```python
from build123d import *

# Parameters (mm, degrees)
SKETCH1_R           = 3
BOSS_EXTRUDE1_DEPTH = 101.6
BOSS_EXTRUDE2_START = 3.175
SKETCH3_R           = 1.0795
BOSS_EXTRUDE2_DEPTH = 3.175


with BuildPart() as part:
    # Sketch1 → Boss-Extrude1 (new body)
    with BuildSketch(Plane(origin=(0, 0, 0), x_dir=(1, 0, 0), z_dir=(0, 1, 0))):
        with Locations(Location((0, 0, 0), (0, 0, 270))):
            Circle(SKETCH1_R)
    extrude(amount=BOSS_EXTRUDE1_DEPTH)

    # Sketch3 → Boss-Extrude2 (add)
    with BuildSketch(Plane.XZ.offset(BOSS_EXTRUDE2_START)):
        with BuildLine():
            Line((-3, 0), (-3, 9.7))
            Line((-3, 9.7), (1.445, 9.7))
            Line((1.445, 9.7), (9.7, 1.445))
            Line((9.7, 1.445), (9.7, -3))
            Line((9.7, -3), (0, -3))
            ThreePointArc((0, -3), (-2.121320344, -2.121320344), (-3, 0))
        make_face()
        with Locations(Location((0.048, 6.34981858, 0), (0, 0, 270))):
            Circle(SKETCH3_R, mode=Mode.SUBTRACT)
        with Locations(Location((6.34981858, 0.048, 0), (0, 0, 270))):
            Circle(SKETCH3_R, mode=Mode.SUBTRACT)
    extrude(amount=-BOSS_EXTRUDE2_DEPTH)


solid = part.part
```
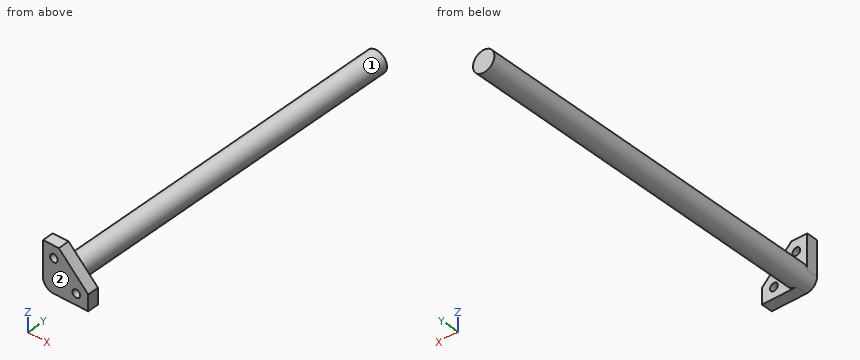
Part model, mm, in its own coordinate system. Face numbers are marked on the shaded views. A direction names the side the tool comes from. Round coordinates to 2 decimals unless told otherwise and drop trailing zeros. Write each loop counter-clockwise with the first axis right and the second up, starting at its lowest first coordinate (ties: lowest second). Pieces come first, ordered by that corner, then holes. Notation, with made-up numbers: M -1,27 L 56,27 A31 ccw 56,51 Z; hole C -11,-1.5 d10. An arc over 180 degrees is marked long. Answer as CSV lines item,"result". Start each with the question number.
1) Band-saw the part on A-A (y = 25.5). List the corners of the cut face in (x, z), then the cut area to 3 significant figures.
2) Drill centre lines: L1, parallel to Y at x = 6.25, z = -2.5 (3 decimals); L2, parallel to Z at x = -0.25, y = 20.5; L3, parallel to X at y = 93, z = 2.5. Where is each one in solid material? Low to high.
3) Which spindle directions (+Z, -Z, +X, -X, +Y, -Y) get a long thin tool onto all of the face, cutting with end or side? Do the marked faces 1 and 2. Say none if no direction does.
4) Band-saw the part on C-C (x = 8.5). List the corners of the cut face in (y, z) (3 decimals), then the cut area to 3 significant figures.
5) Drop flat-ended pins along their axis: pin 1 (6 mm diameter, centred on y = 64, z = 8, fed in from -X); pin 2 (4 mm diameter, centred on x = 7, z = 5, fed in from +Y). Give the stop position or say it passes through.
6) Band-saw the part on B-B (z = 8.5). List the corners of the cut face in (x, y) (3 decimals), then the cut area to 3 significant figures.
Worked out:
1,outline,"C 0,0 d6"
1,area,"28.3 mm²"
2,L1,"-3.175 to 0"
2,L2,"-2.99 to 2.99"
2,L3,"-1.66 to 1.66"
3,face 1,"+Y"
3,face 2,"+Z, -Z, +X, -X, -Y"
4,outline,"M -3.175,-3 L 0,-3 L 0,2.645 L -3.175,2.645 Z"
4,area,"17.9 mm²"
5,pin 1,"through"
5,pin 2,"y = 0"
6,outline,"M -3,-3.175 L 2.645,-3.175 L 2.645,0 L -3,0 Z"
6,area,"17.9 mm²"
